from build123d import *

# Parameters (mm, degrees)
SKETCH1_R           = 65
BOSS_EXTRUDE1_DEPTH = 5
SKETCH2_R           = 10
CUT_EXTRUDE1_DEPTH  = 5
CUT_EXTRUDE3_DEPTH  = 4
CUT_EXTRUDE2_DEPTH  = 93.059763198
BOSS_EXTRUDE2_DEPTH = 11
BOSS_EXTRUDE3_DEPTH = 5
CUT_EXTRUDE4_DEPTH  = 5
CUT_EXTRUDE5_DEPTH  = 2.5
SKETCH16_W          = 21
SKETCH16_H          = 2
BOSS_EXTRUDE5_DEPTH = 4
SKETCH17_W          = 4
SKETCH17_H          = 4
CUT_EXTRUDE8_DEPTH  = 8
BOSS_EXTRUDE6_DEPTH = 6.5
SKETCH23_W          = 64
SKETCH23_H          = 3.5
CUT_EXTRUDE9_DEPTH  = 10


with BuildPart() as part:
    # Sketch1 → Boss-Extrude1 (new body)
    with BuildSketch(Plane(origin=(0, 0, 0), x_dir=(1, 0, 0), z_dir=(0, 1, 0))):
        with Locations(Location((0, 0, 0), (0, 0, 270))):
            Circle(SKETCH1_R)
    extrude(amount=BOSS_EXTRUDE1_DEPTH)

    # Sketch2 → Cut-Extrude1 (cut)
    with BuildSketch(Plane(origin=(0, 5, 0), x_dir=(1, 0, 0), z_dir=(0, 1, 0))):
        with Locations(Location((0, 0, 0), (0, 0, 270))):
            Circle(SKETCH2_R)
    extrude(amount=-CUT_EXTRUDE1_DEPTH, mode=Mode.SUBTRACT)

    # Sketch5 → Cut-Extrude3 (cut)
    with BuildSketch(Plane(origin=(0, 5, 0), x_dir=(1, 0, 0), z_dir=(0, 1, 0))):
        Polygon((0, 47.5), (10.5, 47.5), (10.5, 65), (-10.5, 65), (-10.5, 47.5), align=None)
    extrude(amount=-CUT_EXTRUDE3_DEPTH, mode=Mode.SUBTRACT)

    # Sketch3 → Cut-Extrude2 (cut, through all)
    with BuildSketch(Plane(origin=(0, 5, 0), x_dir=(1, 0, 0), z_dir=(0, 1, 0))):
        with BuildLine():
            Line((43.158190089, -17.309553092), (60.328652813, -24.196149483))
            ThreePointArc((60.328652813, -24.196149483), (63.821479272, -12.321476518), (65, 0))
            ThreePointArc((65, 0), (54.706549574, 35.102612918), (27.086355887, 59.087471809))
            ThreePointArc((27.086355887, 59.087471809), (24.677873317, 60.133206871), (22.229121422, 61.080816635))
            ThreePointArc((22.229121422, 61.080816635), (17.992417486, 62.460170613), (13.671171428, 63.546038994))
            Line((13.671171428, 63.546038994), (12.228525973, 44.863271755))
            ThreePointArc((12.228525973, 44.863271755), (14.077546566, 44.317859636), (15.902371478, 43.696276516))
            ThreePointArc((15.902371478, 43.696276516), (17.654170911, 43.018371069), (19.377162288, 42.270268294))
            ThreePointArc((19.377162288, 42.270268294), (39.136223926, 25.111869241), (46.5, 0))
            ThreePointArc((46.5, 0), (45.656904402, -8.81459474), (43.158190089, -17.309553092))
        make_face()
    extrude(amount=-CUT_EXTRUDE2_DEPTH, mode=Mode.SUBTRACT)

    # Sketch9 → Boss-Extrude2 (add)
    with BuildSketch(Plane.XZ):
        Polygon((-13.753226894, -2.439518395), (-16.581654019, -5.26794552), (-5.26794552, -16.581654019), (-2.439518395, -13.753226894), align=None)
        Polygon((9.899494937, 21.213203436), (7.071067812, 18.384776311), (18.384776311, 7.071067812), (21.213203436, 9.899494937), align=None)
    extrude(amount=BOSS_EXTRUDE2_DEPTH)

    # Sketch10 → Boss-Extrude3 (add)
    with BuildSketch(Plane.XZ.offset(11)):
        Polygon((-5.26794552, -16.581654019), (-16.581654019, -5.26794552), (9.899494937, 21.213203436), (21.213203436, 9.899494937), align=None)
    extrude(amount=BOSS_EXTRUDE3_DEPTH)

    # Sketch11 → Cut-Extrude4 (cut)
    with BuildSketch(Plane.XZ.offset(16)):
        Polygon((6.805902769, 15.467960838), (15.467960838, 6.805902769), (-0.618718434, -9.280776503), (-9.280776503, -0.618718434), align=None)
    extrude(amount=-CUT_EXTRUDE4_DEPTH, mode=Mode.SUBTRACT)

    # Sketch12 → Cut-Extrude5 (cut)
    with BuildSketch(Plane.XZ.offset(16)):
        Polygon((-4.154251265, -12.816309334), (-0.618718434, -9.280776503), (-9.280776503, -0.618718434), (-12.816309334, -4.154251265), align=None)
        Polygon((6.805902769, 15.467960838), (10.3414356, 19.00349367), (19.00349367, 10.3414356), (15.467960838, 6.805902769), align=None)
    extrude(amount=-CUT_EXTRUDE5_DEPTH, mode=Mode.SUBTRACT)

    # Sketch16 → Boss-Extrude5 (add)
    with BuildSketch(Plane(origin=(0, 0, -47.5), x_dir=(-1, 0, 0), z_dir=(0, 0, -1))):
        with Locations((0, 4)):
            Rectangle(SKETCH16_W, SKETCH16_H)
    extrude(amount=BOSS_EXTRUDE5_DEPTH)

    # Sketch17 → Cut-Extrude8 (cut)
    with BuildSketch(Plane(origin=(5.656854249, 0, -5.656854249), x_dir=(-0.7071067811865472, 0, -0.7071067811865479), z_dir=(0.7071067811865479, 0, -0.7071067811865472))):
        with Locations((13.45, -2)):
            Rectangle(SKETCH17_W, SKETCH17_H)
    extrude(amount=-CUT_EXTRUDE8_DEPTH, mode=Mode.SUBTRACT)

    # Sketch22 → Boss-Extrude6 (add)
    with BuildSketch(Plane.XZ):
        Polygon((21.213203436, 9.899494937), (35.355339059, 24.04163056), (42.426406871, 16.970562748), (-7.071067812, -32.526911935), (-14.142135624, -25.455844123), align=None)
    extrude(amount=BOSS_EXTRUDE6_DEPTH)

    # Sketch23 → Cut-Extrude9 (cut)
    with BuildSketch(Plane(origin=(12.727922061, 0, -12.727922061), x_dir=(-0.7071067811865476, 0, -0.7071067811865476), z_dir=(0.7071067811865476, 0, -0.7071067811865476))):
        with Locations((-7, -1.75)):
            Rectangle(SKETCH23_W, SKETCH23_H)
    extrude(amount=-CUT_EXTRUDE9_DEPTH, mode=Mode.SUBTRACT)


solid = part.part
Build history of the part. All positions in model axes, mm. A direction names the side the tool comes from. Round coordinates to 2 decimals unless told otherwise and drop trailing zeros. Order: outer loops, then holes, each group sorted by start corner. A loop starts at its lowest first (then second) coordinate and runs counter-clockwise, first axis right, second up. Notation, with made-up numbers: M -37,53.25 L -27,53.25 A25 cw -27,65.25 Z; hole C 11.5,87 d8. An arc over 180 degrees is marked long. Use CSV: the item, a comma, the result in double quotes. Start each with the question number.
(1) Cut at C-C on x = -30. List the corners of the cut face in (y, z), then the cut area to 3 significant figures.
(2) Cut at B-B on z = 55. List the corners of the cut face in (x, y).
(3) Tool access for faces 1 (the face through (14.612, -14.768, 14.733)), 2 (the face through (28.383, -4.649, 17.07)), 3 (the face through (-8.017, -6.645, -8.176)): list every direction of +Z, -Z, +X, -X, +Y, -Y with a clear straight run to the whole face (end or side of a thin tool).
(4) Cut at A-A on x = 38. List the corners of the cut face in (y, z).
(5) Drill centre lines: probe 1 along Y at (x, z) = (32.5, 17); probe 2 along Y at (x, z) = (19.5, -12.5); probe 3 along Z at (x, y) = (-7, -14.75). Where is each one in solid material? Low to high.
(6) Flat gauge pins, fed straight in: P1, Ø3, axis at x = 7.5, y = -6.5, coming from the -Z side; P2, Ø2, axis at x = 1, y = 4, coming from the -Z side; P3, Ø3, axis at y = 2.5, z = -57.5, coming from the -X side. Where does each tip first touch, or does it go through?
(7) Mould opens along Z. For faces 4 (the face through (-9.76, 2.54, -2.17)), 5 (the face through (19.819, -1.726, 8.505)), 6 (the face through (-4.9, -12.3, -5)), 7 (the face through (38.841, -3.204, 20.556)) say: +Z half, -Z half, draft (parallel to the pull), parting line (faces both ways), or undercut.
Findings:
1,outline,"M 0,-57.66 L 5,-57.66 L 5,57.66 L 0,57.66 Z"
1,area,"577 mm^2"
2,outline,"M -34.64,0 L 34.64,0 L 34.64,5 L -34.64,5 Z"
3,face 1,"-Y"
3,face 2,"+Z, -Y"
3,face 3,"+Z"
4,outline,"M -6.5,12.54 L -3.5,12.54 L -3.5,17.15 L 0,17.15 L 0,-26.8 L 5,-26.8 L 5,52.74 L 0,52.74 L 0,21.4 L -6.5,21.4 Z"
5,probe 1,"y = -6.5 to -3.5, 0 to 5"
5,probe 2,"y = 0 to 5"
5,probe 3,"z = -14.85 to -9.97, 1.66 to 4.31"
6,P1,"stops at z = -19.46"
6,P2,"stops at z = -51.5"
6,P3,"stops at x = -33"
7,face 4,"undercut"
7,face 5,"-Z half"
7,face 6,"undercut"
7,face 7,"+Z half"
